from build123d import *

# Parameters (mm, degrees)
SKETCH1_R           = 4.7625
BOSS_EXTRUDE1_DEPTH = 14.12875
CHAMFER1_SIZE       = 0.254
SKETCH2_R           = 3.2385
CUT_EXTRUDE1_DEPTH  = 29.2575


with BuildPart() as part:
    # Sketch1 → Boss-Extrude1 (new body, symmetric)
    with BuildSketch(Plane(origin=(0, 0, 0), x_dir=(1, 0, 0), z_dir=(0, 1, 0))):
        Circle(SKETCH1_R)
    extrude(amount=BOSS_EXTRUDE1_DEPTH, both=True)

    # Chamfer1
    chamfer1_edges = [part.edges().sort_by_distance(p)[0] for p in [
        (-4.7625, -14.12875, 0),
        (-4.7625, 14.12875, 0),
    ]]
    chamfer(chamfer1_edges, length=CHAMFER1_SIZE)

    # Sketch2 → Cut-Extrude1 (cut, through all)
    with BuildSketch(Plane.XZ.offset(14.12875)):
        Circle(SKETCH2_R)
    extrude(amount=-CUT_EXTRUDE1_DEPTH, mode=Mode.SUBTRACT)


solid = part.part
Read the model definition and answer for the solid it produces. Units are mm, in the model's axes. Round coordinates to 2 decimals unless told otherwise and drop trailing zeros. Loops run counter-clockwise (first coordinate to the right, second up) from the corner with the lowest first, then second, coordinate; pieces in that order, holes last.
Q1. Section C-C on y = -1 is taken. Write down the section's boundary in (x, z) (1 decimal).
Q2. Determine the mould class of faces 1 (the face through (-3.78, 0.19, 2.9)), 2 (the face through (-0.7, -0.2, -3.16)), 3 (the face through (2, -14.129, 3)) for opening direction Z: released by +Z, released by -Z, zero draft, split by the parting line, or undercut.
Q3. Section B-B on z = 0 is taken. Write down the section's boundary in (x, y).
Q4. Each of these flat-tipped pins is pushed along its axis until it touches: pin 1 (5 mm diameter, centred on x = 0, z = 0, fed in from +Y); pin 2 (5 mm diameter, centred on x = -3.5, y = -11, fed in from -Z); pin 3 (5 mm diameter, centred on x = 0.5, z = 1.5, fed in from -Y); pin 4 (1 mm diameter, centred on y = -1, z = 3, fed in from -X). Where does it stop, or does it pass through?
Q5. Consider probe 1 along Z at (x, y) = (0, -3.75); probe 2 along X at (y, z) = (13, -1.75); probe 3 along X at (y, z) = (-1, -0.75). Determine where each line is inside the solid, lowest interval first.
Q6. Section A-A on x = 0 is taken. Write down the section's boundary in (y, z), and give its area (3 significant figures).
Output:
1. outline: circle Ø9.5 at (0, 0); hole circle Ø6.5 at (0, 0)
2. face 1: split by the parting line
2. face 2: undercut
2. face 3: zero draft
3. outline: (-4.76, -13.87) - (-4.51, -14.13) - (-3.24, -14.13) - (-3.24, 14.13) - (-4.51, 14.13) - (-4.76, 13.87) - close; (3.24, -14.13) - (4.51, -14.13) - (4.76, -13.87) - (4.76, 13.87) - (4.51, 14.13) - (3.24, 14.13) - close
4. pin 1: passes through
4. pin 2: stops at z = -4.66
4. pin 3: stops at y = -14.13
4. pin 4: stops at x = -4.05
5. probe 1: z = -4.76 to -3.24, 3.24 to 4.76
5. probe 2: x = -4.43 to -2.72, 2.72 to 4.43
5. probe 3: x = -4.7 to -3.15, 3.15 to 4.7
6. outline: (-14.13, -4.51) - (-13.87, -4.76) - (13.87, -4.76) - (14.13, -4.51) - (14.13, -3.24) - (-14.13, -3.24) - close; (-14.13, 3.24) - (14.13, 3.24) - (14.13, 4.51) - (13.87, 4.76) - (-13.87, 4.76) - (-14.13, 4.51) - close
6. area: 86.0 mm2
